For this review, take the finished solid that the model builds, in its own axes (mm). Coordinates: 2 decimals unless noted, no trailing zeros. Order: outer loops, then holes, each group sorted by start corner. A loop starts at its lowest first (then second) coordinate and runs counter-clockwise, first axis right, second up. Notation, with made-up numbers: (82.5, 78) -> (125.5, 78) arc R11 ccw to (125.5, 85) -> close; hole circle Ø10 at (-8.75, 17.25). An arc over 180 degrees is marked (long way). Return JSON: item names as keys, results as strings. Group by question number.
Item 1: Draft analysis for pull direction Y (two halves, no side actions). For faces 1 (the flat face through (0, 13, 0)), 2 (the cylindrical face through (-0.195, 21.487, 1.521)), 3 (the cylindrical face through (-15.935, -10.575, 1.521)), 4 (the cylindrical face through (0, 50, 1)), state which applies: +Y half, -Y half, draft (parallel to the pull), parting line (faces both ways), or undercut.
Item 2: Insertion check: pin 1 (1 mm diameter, centred on x = -15.5, z = 2, fed in from -Y). The pin has a flat end and moves straight along its axis. Give the tip position at first contact, or say it passes through.
Item 3: For line 1 along Y through (x, z) = (0, 1.95); line 2 along Y through (x, z) = (-16.5, 1.6); line 3 along Y through (x, z) = (-1, 2.4), list the stretches that pass through material, from the lowest coordinate up.
Item 4: Take a section at A-A (z = 1.6). Write out the cut boundary in (x, y), then the cut area to 3 significant figures.
Item 5: Take a section at B-B (y = -20). Write out the cut boundary in (x, z), then the cut area to 3 significant figures.
Item 6: Take a section at C-C (x = -4.5). Write out the cut boundary in (y, z).
Item 7: Take a section at D-D (y = -10). Write out the cut boundary in (x, z), then the cut area to 3 significant figures.
```python
from build123d import *

# Parameters (mm, degrees)
ESQUISSE1_R             = 50
ESQUISSE1_R_2           = 7
BOSS_EXTRU_1_DEPTH      = 3
ESQUISSE2_R             = 1.5
ENL_V_MAT_EXTRU_1_DEPTH = 71.774289117


with BuildPart() as part:
    # Esquisse1 → Boss.-Extru.1 (new body)
    with BuildSketch(Plane.XY):
        Circle(ESQUISSE1_R)
        Circle(ESQUISSE1_R_2, mode=Mode.SUBTRACT)
    extrude(amount=BOSS_EXTRU_1_DEPTH)

    # Esquisse2 → Enlèv. mat.-Extru.1 (cut, through all)
    with BuildSketch(Plane.XY.offset(3)):
        with BuildLine():
            Line((25, 43.301270189), (25, 0))
            ThreePointArc((25, 0), (0, -25), (-25, 0))
            Line((-25, 0), (-25, 43.301270189))
            ThreePointArc((-25, 43.301270189), (0, -50), (25, 43.301270189))
        make_face()
        with Locations((0, 20)):
            Circle(ESQUISSE2_R)
        with Locations((17.320508076, 10)):
            Circle(ESQUISSE2_R)
        with Locations((17.320508076, -10)):
            Circle(ESQUISSE2_R)
        with Locations((0, -20)):
            Circle(ESQUISSE2_R)
        with Locations((-17.320508076, -10)):
            Circle(ESQUISSE2_R)
        with Locations((-17.320508076, 10)):
            Circle(ESQUISSE2_R)
    extrude(amount=-ENL_V_MAT_EXTRU_1_DEPTH, mode=Mode.SUBTRACT)


solid = part.part
```
Findings below:
{
 "1": {"face 1": "draft", "face 2": "undercut", "face 3": "undercut", "face 4": "+Y half"},
 "2": {"pin 1": "stops at y = -20"},
 "3": {"line 1": "y = -25 to -21.5, -18.5 to -7, 7 to 18.5, 21.5 to 50", "line 2": "y = -18.78 to -11.26, -8.74 to 8.74, 11.26 to 47.2", "line 3": "y = -24.98 to -21.12, -18.88 to -6.93, 6.93 to 18.88, 21.12 to 49.99"},
 "4": {"outline": "(-25, 0) arc R25 ccw to (25, 0) -> (25, 43.3) arc R50 ccw to (-25, 43.3) -> close; hole circle Ø3 at (-17.32, -10); hole circle Ø3 at (-17.32, 10); hole circle Ø14 at (0, 0); hole circle Ø3 at (0, -20); hole circle Ø3 at (0, 20); hole circle Ø3 at (17.32, -10); hole circle Ø3 at (17.32, 10)", "area": "3,180 mm2"},
 "5": {"outline": "(-15, 0) -> (-1.5, 0) -> (-1.5, 3) -> (-15, 3) -> close; (1.5, 0) -> (15, 0) -> (15, 3) -> (1.5, 3) -> close", "area": "81.0 mm2"},
 "6": {"outline": "(-24.59, 0) -> (-5.36, 0) -> (-5.36, 3) -> (-24.59, 3) -> close; (5.36, 0) -> (49.8, 0) -> (49.8, 3) -> (5.36, 3) -> close"},
 "7": {"outline": "(-22.91, 0) -> (-18.82, 0) -> (-18.82, 3) -> (-22.91, 3) -> close; (-15.82, 0) -> (15.82, 0) -> (15.82, 3) -> (-15.82, 3) -> close; (18.82, 0) -> (22.91, 0) -> (22.91, 3) -> (18.82, 3) -> close", "area": "119 mm2"}
}
